Part model, mm, in its own coordinate system. Face numbers are marked on the shaded views. Round coordinates to 2 decimals unless told otherwise and drop trailing zeros. Loops run counter-clockwise (first coordinate to the right, second up) from the corner with the lowest first, then second, coordinate; pieces in that order, holes last. Notation, with made-up numbers: M 40,39.25 L 45,39.25 A28 ccw 45,71.25 Z; hole C 18.25,52.5 d4. An arc over 180 degrees is marked long. Write each question's results on one line, items separated by ' | '.
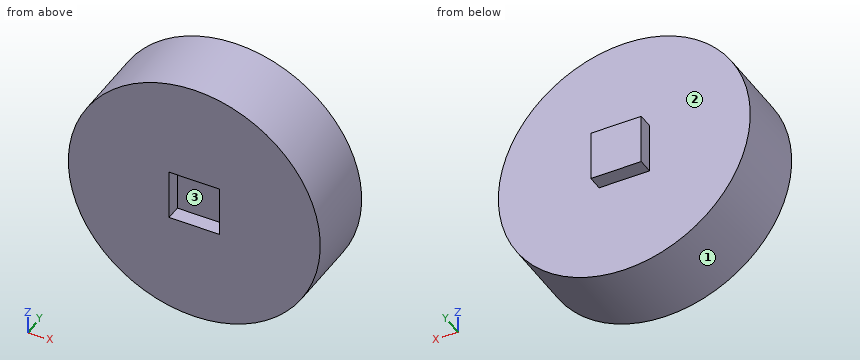
from build123d import *

# Parameters (mm, degrees)
SKETCH1_R           = 25
BOSS_EXTRUDE1_DEPTH = 15
SKETCH2_W           = 10
SKETCH2_H           = 10
BOSS_EXTRUDE2_DEPTH = 3
SKETCH3_W           = 10
SKETCH3_H           = 10
CUT_EXTRUDE1_DEPTH  = 3


with BuildPart() as part:
    # Sketch1 → Boss-Extrude1 (new body)
    with BuildSketch(Plane(origin=(0, 0, 0), x_dir=(1, 0, 0), z_dir=(0, 1, 0))):
        with Locations(Location((0, 0, 0), (0, 0, 270))):
            Circle(SKETCH1_R)
    extrude(amount=BOSS_EXTRUDE1_DEPTH)

    # Sketch2 → Boss-Extrude2 (add)
    with BuildSketch(Plane(origin=(0, 15, 0), x_dir=(1, 0, 0), z_dir=(0, 1, 0))):
        Rectangle(SKETCH2_W, SKETCH2_H)
    extrude(amount=BOSS_EXTRUDE2_DEPTH)

    # Sketch3 → Cut-Extrude1 (cut)
    with BuildSketch(Plane.XZ):
        Rectangle(SKETCH3_W, SKETCH3_H)
    extrude(amount=-CUT_EXTRUDE1_DEPTH, mode=Mode.SUBTRACT)


solid = part.part
Item 1: Band-saw the part on B-B on x = 0. Give the cut face in (y, z), and give its area (3 significant figures).
Filled sheet:
outline: M 0,-25 L 15,-25 L 15,-5 L 18,-5 L 18,5 L 15,5 L 15,25 L 0,25 L 0,5 L 3,5 L 3,-5 L 0,-5 Z | area: 750 mm^2
Item 2: Two-plate mould, pull along Z, no slides. Class the marked faces 1, 2 and 3: +Z half, -Z half, draft (parallel to the pull), parting line (faces both ways), or undercut.
Filled sheet:
face 1: parting line | face 2: draft | face 3: undercut
Item 3: Drop flat-ended pins along their axis: P1, Ø2.5, axis at y = 16, z = 1, coming from the -X side; P2, Ø5, axis at x = 5, y = 10.5, coming from the -Z side; P3, Ø1, axis at x = -6.5, y = 9, coming from the +Z side. Give the stop position or say it passes through.
Filled sheet:
P1: x = -25 | P2: z = -24.87 | P3: z = 24.27
Item 4: Band-saw the part on A-A on y = 2. Give the cut face in (x, z).
Filled sheet:
outline: C 0,0 d50; hole M -5,-5 L 5,-5 L 5,5 L -5,5 Z
Item 5: Band-saw the part on D-D on y = 16. Give the cut face in (x, z), and give its area (3 significant figures).
Filled sheet:
outline: M -5,-5 L 5,-5 L 5,5 L -5,5 Z | area: 100 mm^2
Item 6: Band-saw the part on C-C on z = 0. Give the cut face in (x, y).
Filled sheet:
outline: M -25,0 L -5,0 L -5,3 L 5,3 L 5,0 L 25,0 L 25,15 L 5,15 L 5,18 L -5,18 L -5,15 L -25,15 Z
Item 7: Wall check: L1, parallel to Z at x = -0.5, y = 9.5 (3 decimals); L2, parallel to Y at x = -21, z = 5; L3, parallel to X at y = 16.25, z = 4.5. Give the ranges that are in metal, low to high.
Filled sheet:
L1: -24.995 to 24.995 | L2: 0 to 15 | L3: -5 to 5
